Can you work these out from the model? Positions are in its coordinate system, mm. Coordinates: 2 decimals unless noted, no trailing zeros. Order: outer loops, then holes, each group sorted by start corner. A loop starts at its lowest first (then second) coordinate and runs counter-clockwise, first axis right, second up. Notation, with made-up numbers: (-12, 10.5) -> (6, 10.5) arc R28 cw to (6, 34.5) -> close; hole circle Ø10 at (-34, 19). An arc over 180 degrees is marked (long way). Answer in a Markdown table with one row per item. Add a question column.
1. Imagine slicing it at A-A on z = -7.75. Write out the boundary of the cut face in (x, y), plus the area to 3 significant figures.
2. Will these pins go through, and if not, where does the flat tip stop? pin 1 (4 mm diameter, centred on x = 10.5, z = -5, fed in from +Y); pin 2 (6 mm diameter, centred on x = -7.5, z = -5.5, fed in from -Y).
3. If I drill on line 1 along X through (y, z) = (0, -6.75); line 2 along X through (y, z) = (-7.5, -7.75); line 3 along Y through (x, z) = (-4.75, -9), over which ranges is the centre line in solid material (lowest first)? Write a range as [from, to].
Autodesk Inventor part; units mm, degrees
ref_plane "NUT_XY" through (0, 0, 0) normal (0, 0, 1) x (1, 0, 0)
ref_plane "NUT_YZ" through (0, 0, 0) normal (1, 0, 0) x (0, 1, 0)
ref_plane "NUT_ZX" through (0, 0, 0) normal (0, 1, 0) x (0, 0, 1)
sketch "Sketch_8" plane through (0, 0, 0) normal (1, 0, 0) x (0, 1, 0)
  line L0 (0, -10.668) -> (0, 0)
  line L1 (0, 0) -> (14.224, 0)
  line L2 (14.224, 0) -> (17.0688, -0.7623)
  line L3 (17.0688, -0.7623) -> (17.0688, -9.9057)
  line L4 (17.0688, -9.9057) -> (14.224, -10.668)
  line L5 (14.224, -10.668) -> (0, -10.668)
  line L6 (0, -10.668) -> (0, 0)
sketch "Sketch_10" plane through (0, 0, 0) normal (0, 0, 1) x (1, 0, 0)
  line L0 (-28.448, -28.448) -> (28.448, -28.448)
  line L1 (28.448, -28.448) -> (28.448, 28.448)
  line L2 (28.448, 28.448) -> (-28.448, 28.448)
  line L3 (-28.448, 28.448) -> (-28.448, -28.448)
  line L4 (-14.224, -8.2122) -> (0, -16.4245)
  line L5 (0, -16.4245) -> (14.224, -8.2122)
  line L6 (14.224, -8.2122) -> (14.224, 8.2122)
  line L7 (14.224, 8.2122) -> (0, 16.4245)
  line L8 (0, 16.4245) -> (-14.224, 8.2122)
  line L9 (-14.224, 8.2122) -> (-14.224, -8.2122)
revolve "Revolution1" add sketch "Sketch_8" angle 360 about axis through (0, 0, -10.668) along (0, 0, -1)
extrude "Extrusion1" cut sketch "Sketch_10" against normal blind 10.668
sketch "Sketch_11" plane through (0, 0, 0) normal (1, 0, 0) x (0, 1, 0)
  line L0 (0, -10.668) -> (0, 0)
  line L1 (0, 0) -> (9.525, 0)
  line L2 (9.525, 0) -> (8.6652, -0.8598)
  line L3 (8.6652, -0.8598) -> (8.6652, -9.8082)
  line L4 (8.6652, -9.8082) -> (9.525, -10.668)
  line L5 (9.525, -10.668) -> (0, -10.668)
  line L6 (0, -10.668) -> (0, 0)
revolve "Revolution2" cut sketch "Sketch_11" angle 360 about axis through (0, 0, -10.668) along (0, 0, -1)
thread "Thread1"
ref_plane "NUT_XY" through (0, 0, 0) normal (0, 0, 1) x (1, 0, 0)
ref_plane "NUT_YZ" through (0, 0, 0) normal (1, 0, 0) x (0, 1, 0)
ref_plane "NUT_ZX" through (0, 0, 0) normal (0, 1, 0) x (0, 0, 1)
ref_plane "a1_XY" through (-14.224, 14.224, 0) normal (0, 0, 1) x (1, 0, 0)
ref_plane "a1_YZ" through (-14.224, 14.224, 0) normal (1, 0, 0) x (0, 1, 0)
ref_plane "a1_ZX" through (-14.224, 14.224, 0) normal (0, 1, 0) x (0, 0, 1)
ref_plane "a2_XY" through (14.224, 14.224, 0) normal (0, 0, 1) x (1, 0, 0)
ref_plane "a2_YZ" through (14.224, 14.224, 0) normal (1, 0, 0) x (0, 1, 0)
ref_plane "a2_ZX" through (14.224, 14.224, 0) normal (0, 1, 0) x (0, 0, 1)
ref_plane "b1_XY" through (0, 14.224, 0) normal (1, 0, 0) x (0, 0, -1)
ref_plane "b1_YZ" through (0, 14.224, 0) normal (0, 0, -1) x (0, 1, 0)
ref_plane "b1_ZX" through (0, 14.224, 0) normal (0, 1, 0) x (1, 0, 0)
ref_plane "b2_XY" through (0, 14.224, -10.668) normal (1, 0, 0) x (0, 0, -1)
ref_plane "b2_YZ" through (0, 14.224, -10.668) normal (0, 0, -1) x (0, 1, 0)
ref_plane "b2_ZX" through (0, 14.224, -10.668) normal (0, 1, 0) x (1, 0, 0)
ref_plane "e_XY" through (0, 0, -10.668) normal (1, 0, 0) x (0, 0, -1)
ref_plane "e_YZ" through (0, 0, -10.668) normal (0, 0, -1) x (0, 1, 0)
ref_plane "e_ZX" through (0, 0, -10.668) normal (0, 1, 0) x (1, 0, 0)
ref_plane "ol1_XY" through (0, 0, -14.224) normal (0, 1, 0) x (1, 0, 0)
ref_plane "ol1_YZ" through (0, 0, -14.224) normal (1, 0, 0) x (0, 0, -1)
ref_plane "ol1_ZX" through (0, 0, -14.224) normal (0, 0, -1) x (0, 1, 0)
ref_plane "ol2_XY" through (10.668, 0, -14.224) normal (0, 1, 0) x (1, 0, 0)
ref_plane "ol2_YZ" through (10.668, 0, -14.224) normal (1, 0, 0) x (0, 0, -1)
ref_plane "ol2_ZX" through (10.668, 0, -14.224) normal (0, 0, -1) x (0, 1, 0)
ref_plane "th1_XY" through (0, 9.525, -10.668) normal (1, 0, 0) x (0, 0, -1)
ref_plane "th1_YZ" through (0, 9.525, -10.668) normal (0, 0, -1) x (0, 1, 0)
ref_plane "th1_ZX" through (0, 9.525, -10.668) normal (0, 1, 0) x (1, 0, 0)
ref_plane "th2_XY" through (0, -9.525, -10.668) normal (1, 0, 0) x (0, 0, -1)
ref_plane "th2_YZ" through (0, -9.525, -10.668) normal (0, 0, -1) x (0, 1, 0)
ref_plane "th2_ZX" through (0, -9.525, -10.668) normal (0, 1, 0) x (1, 0, 0)
properties part number "D-3556"
Answers follow:
| question | item | result |
|---|---|---|
| 1 | outline | (-14.22, -8.21) -> (0, -16.42) -> (14.22, -8.21) -> (14.22, 8.21) -> (0, 16.42) -> (-14.22, 8.21) -> close; hole circle Ø17.33 at (0, 0) |
| 1 | area | 465 mm² |
| 2 | pin 1 | stops at y = 11.52 |
| 2 | pin 2 | stops at y = -13.83 |
| 3 | line 1 | x = [-14.22, -8.67], [8.67, 14.22] |
| 3 | line 2 | x = [-14.22, -4.34], [4.34, 14.22] |
| 3 | line 3 | y = [-13.68, -7.25], [7.25, 13.68] |
